Geometry check sheet. Reference: the model listing, model coordinates, mm. A direction names the side the tool comes from. Give positions to 0.01 mm unless a question says otherwise; leave off trailing zeros. Loops run counter-clockwise (first coordinate to the right, second up) from the corner with the lowest first, then second, coordinate; pieces in that order, holes last. Notation, with made-up numbers: (6, -22.75) - (65, -22.75) arc R22 ccw to (65, -8.75) - close; hole circle Ø7 at (26, 4.5). An arc over 180 degrees is marked (long way). Use a Markdown table: item, result. Add a question column.
1. Cross-section at A-A on x = 303.4. Enter the section's corners in (y, z).
2. Cross-section at D-D on z = -53. Enter the section's corners in (x, y).
3. Cross-section at C-C on z = -11. Enter the section's corners in (x, y), and give its area (3 significant figures).
4. Set-up check for faces 4 (the flat face through (130, 18, -204)), 5 (the flat face through (34, 7, -174)), 6 (the flat face through (195, 35, -36)), 7 (the flat face through (265, 44.5, -322)), 8 (the flat face through (310, 25, -330)): record each of +Z, -Z, +X, -X, +Y, -Y from which the full face is reachable in a straight line by a thin tool's end or side.
5. Depth check by flat-ended pin: P1, Ø15, axis at x = 262, z = -328, coming from the +Y side; P2, Ø11, axis at x = 330.5, y = 44, coming from the -Z side; P3, Ø4, axis at x = 142.5, y = 33, coming from the -Z side. Enter the tip coordinate at first touch or a pass-through.
6. Cross-section at B-B on z = -224.5. Enter the section's corners in (x, y), and give its area (3 significant figures).
7. Material ranges on L1, parallel to Z at x = 265, y = 13; L2, parallel to Z at x = 373, y = 17; L3, parallel to X at y = 14.5, z = -11, recorded low to high.
8. Draft check along X on faces 1 (the flat face through (348, 25, -313)), 2 (the flat face through (221, 32, -123)), 3 (the flat face through (48, 19, -15)). Enter one of: pulls with the +X half, pulls with the -X half, needs draft (parallel to the pull), parting line crosses it, or undercut.
Autodesk Inventor part; units mm, degrees
ref_plane "YZ Plane" through (0, 0, 0) normal (1, 0, 0) x (0, 1, 0)
ref_plane "XZ Plane" through (0, 0, 0) normal (0, 1, 0) x (-1, 0, 0)
ref_plane "XY Plane" through (0, 0, 0) normal (0, 0, 1) x (1, 0, 0)
sketch "Sketch1" plane through (0, 0, 0) normal (0, 1, 0) x (-1, 0, 0)
  line L0 (0, 0) -> (-384, 0)
  line L1 (-384, 0) -> (-384, -343)
  line L2 (-384, -343) -> (0, -343)
  line L3 (0, -343) -> (0, 0)
  dimension "d0" = 384
  dimension "d1" = 343
extrude "Extrusion1" add sketch "Sketch1" along normal blind 48.5
sketch "Sketch3" plane through (384, 0, 0) normal (1, 0, 0) x (0, 0, -1)
  line L0 (0, 0) -> (343, 0)
  line L1 (0, 0) -> (0, 48.5)
  line L2 (343, 0) -> (343, 48.5)
  line L3 (30, 48.5) -> (65, 48.5)
  line L4 (30, 48.5) -> (30, 37)
  line L5 (65, 48.5) -> (74.6496, 37)
  line L6 (43, 37) -> (74.6496, 37)
  line L7 (30, 37) -> (30, 35)
  line L8 (30, 35) -> (43, 35)
  line L9 (43, 35) -> (43, 37)
  dimension "d23" = 35
  dimension "d37" = 2
  dimension "d38" = 13
extrude "Extrusion2" cut sketch "Sketch3" against normal through all
sketch "Sketch7" plane through (384, 0, 0) normal (1, 0, 0) x (0, 0, -1)
  line L0 (65, 48.5) -> (343, 48.5)
  line L1 (65, 48.5) -> (161, 48.5)
  line L2 (161, 48.5) -> (174.2196, 48.5) construction
  line L3 (161, 48.5) -> (205, 48.5)
  line L4 (0, 0) -> (343, 0)
  line L5 (151.3504, 37) -> (192, 37)
  line L6 (205, 37) -> (205, 48.5)
  line L7 (161, 48.5) -> (151.3504, 37)
  line L8 (161, 48.5) -> (183.0653, 48.5) construction
  line L9 (205, 37) -> (205, 35)
  line L10 (205, 35) -> (192, 35)
  line L11 (192, 35) -> (192, 37)
  dimension "d27" = 96
  dimension "d29" = 44
  dimension "d32" = 130
extrude "Extrusion3" cut sketch "Sketch7" against normal through all
sketch "Sketch8" plane through (0, 48.5, 0) normal (0, 1, 0) x (1, 0, 0)
  line L0 (310, 343) -> (310, 316)
  line L1 (313, 313) -> (384, 313)
  line L2 (384, 0) -> (384, 343)
  line L3 (384, 313) -> (384, 343)
  line L4 (384, 343) -> (310, 343)
  line L5 (384, 343) -> (0, 343)
  arc A0 (310, 316) -> (313, 313) centre (313, 316) ccw
  point P0 (0, 0)
  point P1 (310, 313)
  dimension "d43" = 30
  dimension "d46" = 3
extrude "Extrusion4" cut sketch "Sketch8" against normal through all
sketch "Sketch9" plane through (0, 0, -343) normal (0, 0, -1) x (-1, 0, 0)
  line L0 (-215, 7) -> (-225, 7)
  line L1 (-255, 7) -> (-255, 0)
  line L2 (-255, 7) -> (-240, 24.8763)
  line L3 (-225, 7) -> (-240, 24.8763)
  line L4 (-215, 7) -> (-215, 0)
  line L5 (-255, 0) -> (-215, 0)
  dimension "d50" = 10
extrude "Extrusion5" cut sketch "Sketch9" against normal through all
sketch "Sketch10" plane through (0, 48.5, 0) normal (0, 1, 0) x (1, 0, 0)
  line L0 (215, 343) -> (215, 0)
  line L1 (215, 343) -> (215, 0)
  line L2 (310, 343) -> (0, 343)
  line L3 (384, 151.3504) -> (0, 151.3504)
  line L4 (215, 343) -> (48, 343)
  line L5 (48, 343) -> (48, 204)
  line L6 (48, 204) -> (215, 204)
  line L7 (215, 204) -> (215, 343)
  point P0 (0, 0)
  dimension "d58" = 167
  dimension "d59" = 139
extrude "Extrusion6" cut sketch "Sketch10" against normal through all
sketch "Sketch11" plane through (0, 0, -343) normal (0, 0, -1) x (-1, 0, 0)
  line L0 (-20, 0) -> (-20, 7)
  line L1 (-20, 7) -> (-48, 7)
  line L2 (-48, 0) -> (-48, 7)
  line L3 (-48, 0) -> (-20, 0)
  dimension "d65" = 7
extrude "Extrusion7" cut sketch "Sketch11" against normal through all
sketch "Sketch12" plane through (0, 48.5, 0) normal (0, 1, 0) x (1, 0, 0)
  line L0 (221, 113) -> (221, 128)
  line L1 (211, 88) -> (0, 88)
  line L2 (211, 138) -> (0, 138)
  arc A0 (211, 88) -> (221, 98) centre (211, 98) ccw
  arc A1 (221, 128) -> (211, 138) centre (211, 128) ccw
  line L3 (221, 98) -> (221, 113)
  line L4 (0, 88) -> (0, 138)
  point P0 (384, 161)
  point P1 (221, 88)
  dimension "d72" = 10
extrude "Extrusion8" cut sketch "Sketch12" against normal blind 33
sketch "Sketch14" plane through (384, 0, 0) normal (1, 0, 0) x (0, 0, -1)
  circle A0 centre (109.1034, 31.5) radius 13.5
  line L0 (65, 48.5) -> (161, 48.5)
  point P0 (0, 0)
  dimension "d92" = 27
  dimension "d97" = 17
extrude "Extrusion10" cut sketch "Sketch14" against normal through all
sketch "Sketch17" plane through (0, 0, -343) normal (0, 0, -1) x (-1, 0, 0)
  line L0 (-23, 48.5) -> (-48, 32.2648)
  line L1 (-211, 15.5) -> (0, 15.5)
  line L2 (-48, 35) -> (-48, 7)
  line L3 (-48, 32.2648) -> (-48, 48.5)
  line L4 (-23, 48.5) -> (-48, 48.5)
  point P0 (0, 0)
  point P1 (0, 48.5)
  dimension "d98" = 23
extrude "Extrusion11" cut sketch "Sketch17" against normal up to surface (138 mm away)
sketch "Sketch19" plane through (310, 0, -343) normal (0, 0, -1) x (-1, 0, 0)
  line L0 (0, 48.5) -> (0, 0)
  line L1 (55, 46.5) -> (74.3713, 46.5) construction
  line L2 (55, 46.5) -> (95, 21.5052)
  line L3 (55, 46.5) -> (104.9882, 46.5) construction
  line L4 (55, 46.5) -> (55, 48.5)
  line L5 (55, 48.5) -> (95, 48.5)
  line L6 (89, 48.5) -> (99, 48.5)
  line L7 (95, 48.5) -> (95, 21.5052)
  line L8 (95, 7) -> (95, 48.5)
  point P0 (310, 0)
  dimension "d109" = 32
extrude "Extrusion12" cut sketch "Sketch19" against normal up to surface (138 mm away)
sketch "Sketch25" plane through (0, 48.5, 0) normal (0, 1, 0) x (1, 0, 0)
  arc A0 (310, 316) -> (313, 313) centre (313, 316) ccw
  line L0 (265.5, 314) -> (255, 314)
  line L1 (255, 343) -> (255, 0)
  line L2 (310, 343) -> (255, 343)
  line L3 (280, 328.5) -> (280, 343)
  arc A1 (265.5, 314) -> (280, 328.5) centre (265.5, 328.5) ccw
  line L4 (280, 343) -> (255, 343)
  line L5 (255, 314) -> (255, 343)
  point P0 (0, 0)
extrude "Extrusion16" cut sketch "Sketch25" against normal blind 2
sketch "Sketch26" plane through (0, 46.5, 0) normal (0, 1, 0) x (1, 0, 0)
  line L0 (280, 343) -> (280, 328.5)
  circle A0 centre (265.5, 328.5) radius 9.5
  point P0 (0, 0)
  dimension "d136" = 19
extrude "Extrusion17" cut sketch "Sketch26" against normal blind 2
sketch "Sketch27" plane through (265.5, 44.5, -328.5) normal (0, 1, 0) x (1, 0, 0)
  circle A0 centre (0, 0) radius 6
  point P0 (-265.5, -328.5)
  dimension "d139" = 12
extrude "Extrusion18" cut sketch "Sketch27" against normal through all
sketch "Sketch28" plane through (0, 48.5, 0) normal (0, 1, 0) x (1, 0, 0)
  circle A0 centre (373, 302) radius 5.8
  circle A1 centre (303.4, 302) radius 5.8
  circle A2 centre (373, 11) radius 5.8
  circle A3 centre (303.4, 11) radius 5.8
  point P0 (0, 0)
  point P1 (384, 313)
  point P2 (384, 0)
  dimension "d146" = 11.6
  dimension "d149" = 11.6
  dimension "d152" = 11.6
  dimension "d155" = 11.6
extrude "Extrusion19" cut sketch "Sketch28" against normal through all
sketch "Sketch29" plane through (0, 48.5, 0) normal (0, 0, 1) x (1, 0, 0)
  line L0 (0, -48.5) -> (0, 0)
  line L1 (0, 0) -> (384, 0)
  line L2 (23, 0) -> (48, -16.2352)
  line L3 (23, 0) -> (48, -16.2352)
  line L4 (48, -48.5) -> (215, -48.5)
  line L5 (23, 0) -> (48, 0)
  line L6 (48, -16.2352) -> (48, 0)
  line L7 (384, -13.5) -> (0, -13.5)
extrude "Extrusion20" cut sketch "Sketch29" against normal up to surface (30 mm away) contours L7 L6 L2 | L2 L1 L6 L7
sketch "Sketch30" plane through (0, 0, 0) normal (0, 0, 1) x (1, 0, 0)
  line L0 (48, 48.5) -> (215, 48.5)
  line L1 (215, 48.5) -> (215, 0)
  line L2 (215, 0) -> (48, 0)
  line L3 (48, 0) -> (48, 48.5)
  point P0 (0, 0)
extrude "Extrusion21" cut sketch "Sketch30" against normal up to surface (30 mm away)
sketch "Sketch32" plane through (0, 48.5, 0) normal (0, 1, 0) x (1, 0, 0)
  line L0 (275, 266) -> (283, 266) construction
  circle A0 centre (280.6569, 260.3431) radius 8
  point P0 (0, 0)
  point P1 (255, 343)
  dimension "d168" = 16
extrude "Extrusion22" cut sketch "Sketch32" against normal blind 10
properties part number "saddle"
Values found:
| question | item | result |
|---|---|---|
| 1 | outline | (0, -343) - (48.5, -343) - (48.5, -307.8) - (0, -307.8) - close; (0, -296.2) - (48.5, -296.2) - (48.5, -205) - (35, -205) - (35, -192) - (37, -192) - (37, -151.35) - (48.5, -161) - (48.5, -65) - (37, -74.65) - (37, -43) - (35, -43) - (35, -30) - (48.5, -30) - (48.5, -16.8) - (0, -16.8) - close; (0, -5.2) - (48.5, -5.2) - (48.5, 0) - (0, 0) - close; hole circle Ø27 at (31.5, -109.1) |
| 2 | outline | (0, 0) - (20, 0) - (20, 7) - (48, 7) - (48, 0) - (215, 0) - (215, 7) - (225, 7) - (240, 24.88) - (255, 7) - (255, 0) - (384, 0) - (384, 37) - (0, 37) - close |
| 3 | outline | (0, 0) - (20, 0) - (20, 7) - (48, 7) - (48, 32.26) - (23, 48.5) - (0, 48.5) - close; (215, 7) - (225, 7) - (240, 24.88) - (255, 7) - (255, 0) - (297.6, 0) - (297.6, 48.5) - (215, 48.5) - close; (309.2, 0) - (367.2, 0) - (367.2, 48.5) - (309.2, 48.5) - close; (378.8, 0) - (384, 0) - (384, 48.5) - (378.8, 48.5) - close |
| 3 | area | 8,450 mm2 |
| 4 | face 4 | -Z, +Y, -Y |
| 4 | face 5 | +Z, -Z, -Y |
| 4 | face 6 | +X, -X, +Y |
| 4 | face 7 | +Y |
| 4 | face 8 | -Z, +X, +Y, -Y |
| 5 | P1 | stops at y = 46.5 |
| 5 | P2 | stops at z = -313 |
| 5 | P3 | stops at z = -204 |
| 6 | outline | (0, 0) - (20, 0) - (20, 7) - (48, 7) - (48, 32.26) - (23, 48.5) - (0, 48.5) - close; (215, 7) - (225, 7) - (240, 24.88) - (255, 7) - (255, 0) - (384, 0) - (384, 48.5) - (255, 48.5) - (255, 46.5) - (215, 21.51) - close |
| 6 | area | 9,000 mm2 |
| 7 | L1 | z = -343 to -334.48, -322.52 to 0 |
| 7 | L2 | z = -313 to -307.8, -296.2 to -16.8, -5.2 to 0 |
| 7 | L3 | x = 0 to 48, 215 to 231.29, 248.71 to 297.6, 309.2 to 367.2, 378.8 to 384 |
| 8 | face 1 | needs draft |
| 8 | face 2 | pulls with the -X half |
| 8 | face 3 | undercut |
